Model file for the job. Use its own axes, mm. A direction names the side the tool comes from. Round coordinates to 2 decimals unless told otherwise and drop trailing zeros. Order: outer loops, then holes, each group sorted by start corner. A loop starts at its lowest first (then second) coordinate and runs counter-clockwise, first axis right, second up. Notation, with made-up numbers: M 64,78.25 L 102,78.25 A18 ccw 102,99.25 Z; hole C 20.5,-35 d2. An arc over 180 degrees is marked long. Return JSON: item names as keys, results as strings. Group by question number.
Item 1: Probe line 1 along Z through (x, y) = (0, 27.3); line 2 along Z through (x, y) = (10.5, 22). List the from-to ranges inside material, lowest first.
Item 2: Which spindle directions (+Z, -Z, +X, -X, +Y, -Y) get a long thin tool onto all of the face, cutting with end or side? Do faces 4 (the face through (-14, 0, -14)), 5 (the face through (-7.5, 12, 14)), 6 (the face through (14, 12, 7.5)). Say none if no direction does.
Item 3: Slice it at D-D on x = -12. Write the cut outline in (y, z), then the cut area to 3 significant figures.
Item 4: Pin check, flat tips, straight feed: pin 1 Ø8 at (x, y) = (-1, 20) entering from -Z; pin 2 Ø5 at (x, z) = (4.5, -3) entering from -Y. Stop position of each tip, or through.
Item 5: Slice it at A-A on x = 0. Write the cut outline in (y, z).
Item 6: Pull direction X, two halves, no side cores. Call faces 1 (the face through (14, 12, -7.5)), 2 (the face through (7.5, 12, -14)), 3 (the face through (-18, 15, -19)): pulls with the +X half, pulls with the -X half, needs draft (parallel to the pull), parting line crosses it, or undercut.
Item 7: Slice it at B-B on z = -10. Write the cut outline in (x, y), then the cut area to 3 significant figures.
Item 8: Slice it at C-C on y = 9.25. Write the cut outline in (x, z).
from build123d import *

# Parameters (mm, degrees)
SKIZZE1_W                       = 40
SKIZZE1_H                       = 40
AUFSATZ_LINEAR_AUSTRAGEN1_DEPTH = 30
FASE1_SIZE                      = 3
SCHNITT_LINEAR_AUSTRAGEN1_DEPTH = 25
DURCHGANGSLOCH_F_R_M31_D        = 3.2


with BuildPart() as part:
    # Skizze1 → Aufsatz-Linear austragen1 (new body)
    with BuildSketch(Plane(origin=(0, 0, 0), x_dir=(1, 0, 0), z_dir=(0, 1, 0))):
        Rectangle(SKIZZE1_W, SKIZZE1_H)
    extrude(amount=AUFSATZ_LINEAR_AUSTRAGEN1_DEPTH)

    # Fase1
    fase1_edges = [part.edges().sort_by_distance(p)[0] for p in [
        (-20, 15, -20),
        (20, 15, -20),
        (20, 15, 20),
        (-20, 15, 20),
    ]]
    chamfer(fase1_edges, length=FASE1_SIZE)

    # Skizze2 → Schnitt-Linear austragen1 (cut)
    with BuildSketch(Plane.XZ):
        Polygon((-20, 7.5), (-7.5, 7.5), (-7.5, 20), (7.5, 20), (7.5, 7.5), (20, 7.5), (20, -7.5), (7.5, -7.5), (7.5, -20), (-7.5, -20), (-7.5, -7.5), (-20, -7.5), align=None)
    extrude(amount=-SCHNITT_LINEAR_AUSTRAGEN1_DEPTH, mode=Mode.SUBTRACT)

    # Durchgangsloch für M31 (through all)
    with Locations(Plane(origin=(0, 30, 0), x_dir=(1, 0, 0), z_dir=(0, 1, 0))):
        with Locations((0, 10), (0, -10)):
            Hole(DURCHGANGSLOCH_F_R_M31_D / 2)


solid = part.part
Output values:
{
 "1": {"line 1": "-20 to -11.6, -8.4 to 8.4, 11.6 to 20", "line 2": "-20 to -7.5, 7.5 to 20"},
 "2": {"face 4": "+Z, -Z, +X, -X, -Y", "face 5": "+Z, -Z, -Y", "face 6": "+X, -X, -Y"},
 "3": {"outline": "M 0,-20 L 30,-20 L 30,20 L 0,20 L 0,7.5 L 25,7.5 L 25,-7.5 L 0,-7.5 Z", "area": "825 mm²"},
 "4": {"pin 1": "through", "pin 2": "y = 25"},
 "5": {"outline": "M 25,-20 L 30,-20 L 30,-11.6 L 25,-11.6 Z; M 25,-8.4 L 30,-8.4 L 30,8.4 L 25,8.4 Z; M 25,11.6 L 30,11.6 L 30,20 L 25,20 Z"},
 "6": {"face 1": "needs draft", "face 2": "undercut", "face 3": "pulls with the -X half"},
 "7": {"outline": "M -20,0 L -7.5,0 L -7.5,25 L -1.6,25 L -1.6,30 L -20,30 Z; M 1.6,25 L 7.5,25 L 7.5,0 L 20,0 L 20,30 L 1.6,30 Z", "area": "809 mm²"},
 "8": {"outline": "M -20,-17 L -17,-20 L -7.5,-20 L -7.5,-7.5 L -20,-7.5 Z; M -20,7.5 L -7.5,7.5 L -7.5,20 L -17,20 L -20,17 Z; M 7.5,-20 L 17,-20 L 20,-17 L 20,-7.5 L 7.5,-7.5 Z; M 7.5,7.5 L 20,7.5 L 20,17 L 17,20 L 7.5,20 Z"}
}
